```python
from build123d import *

# Parameters (mm, degrees)
SKETCH1_R           = 1.699999809
SKETCH1_R_2         = 1.70000044
BOSS_EXTRUDE1_DEPTH = 5
CHAMFER1_SIZE       = 1.5


with BuildPart() as part:
    # Sketch1 → Boss-Extrude1 (new body)
    with BuildSketch(Plane.XY):
        with BuildLine():
            Line((34.170001984, 18.130024456), (34.170001984, 8.129999593))
            ThreePointArc((34.170001984, 8.129999593), (31.826856233, 2.473145343), (26.170001984, 0.129999593))
            Line((26.170001984, 0.129999593), (8.170027525, 0.129999593))
            ThreePointArc((8.170027525, 0.129999593), (2.513173276, 2.473145343), (0.170027525, 8.129999593))
            Line((0.170027525, 8.129999593), (0.170027525, 18.130024456))
            ThreePointArc((0.170027525, 18.130024456), (2.513173276, 23.786878706), (8.170027525, 26.130024456))
            Line((8.170027525, 26.130024456), (26.170001984, 26.130024456))
            ThreePointArc((26.170001984, 26.130024456), (31.826856233, 23.786878706), (34.170001984, 18.130024456))
        make_face()
        with Locations((17.17000103, 3.630000114)):
            Circle(SKETCH1_R, mode=Mode.SUBTRACT)
        with Locations((17.170001507, 22.630000114)):
            Circle(SKETCH1_R_2, mode=Mode.SUBTRACT)
        with BuildLine():
            Line((30.170001984, 15.629999161), (29.170001984, 15.629999161))
            ThreePointArc((29.170001984, 15.629999161), (28.816448593, 15.77644577), (28.670001984, 16.129999161))
            Line((28.670001984, 16.129999161), (28.670001984, 18.879999161))
            ThreePointArc((28.670001984, 18.879999161), (28.523555374, 19.233552551), (28.170001984, 19.379999161))
            Line((28.170001984, 19.379999161), (6.17000103, 19.379999161))
            ThreePointArc((6.17000103, 19.379999161), (5.816447639, 19.233552551), (5.67000103, 18.879999161))
            Line((5.67000103, 18.879999161), (5.67000103, 7.379999638))
            ThreePointArc((5.67000103, 7.379999638), (5.816447639, 7.026446247), (6.17000103, 6.879999638))
            Line((6.17000103, 6.879999638), (28.170001984, 6.879999638))
            ThreePointArc((28.170001984, 6.879999638), (28.523555374, 7.026446247), (28.670001984, 7.379999638))
            Line((28.670001984, 7.379999638), (28.670001984, 10.130000114))
            ThreePointArc((28.670001984, 10.130000114), (28.816448593, 10.483553505), (29.170001984, 10.630000114))
            Line((29.170001984, 10.630000114), (30.170001984, 10.630000114))
            ThreePointArc((30.170001984, 10.630000114), (30.523555374, 10.776446724), (30.670001984, 11.130000114))
            Line((30.670001984, 11.130000114), (30.670001984, 15.129999161))
            ThreePointArc((30.670001984, 15.129999161), (30.523555374, 15.483552551), (30.170001984, 15.629999161))
        make_face(mode=Mode.SUBTRACT)
    extrude(amount=BOSS_EXTRUDE1_DEPTH)

    # Chamfer1
    chamfer1_edges = [part.edges().sort_by_distance(p)[0] for p in [
        (15.470001221, 3.630000114, 5),
        (15.470001067, 22.630000114, 5),
    ]]
    chamfer(chamfer1_edges, length=CHAMFER1_SIZE)


solid = part.part
```
CAD build for the part. Positions are in the model's coordinates, mm. A direction names the side the tool comes from. Coordinates: 2 decimals unless noted, no trailing zeros. Order: outer loops, then holes, each group sorted by start corner. A loop starts at its lowest first (then second) coordinate and runs counter-clockwise, first axis right, second up. Notation, with made-up numbers: M -1,-3 L 10,-3 A21 cw 10,4 Z; hole C -15,-21 d8. An arc over 180 degrees is marked long. Write each question's results on one line, items separated by ' | '. Start each with the question number.
Q1. Drill centre lines: probe 1 along Y at (x, z) = (20, 2.85); probe 2 along X at (y, z) = (8.75, 0.95); probe 3 along Y at (x, z) = (16.5, 4.2). Where is each one in solid material? Low to high. Write a range as from..to.
Q2. Cut at D-D (z = 2.75). List the corners of the cut face in (x, y), then the cut area to 3 significant figures.
Q3. Cut at A-A (x = 9). List the corners of the cut face in (y, z), then the cut area to 3 significant figures.
Q4. Cut at B-B (y = 22.63). List the corners of the cut face in (x, z).
Q5. Cut at C-C (z = 4.3). List the corners of the cut face in (x, y).
Q6. Which spindle directions (+Z, -Z, +X, -X, +Y, -Y) get a long thin tool onto all of the face, cutting with end or side? Do faces 1 (the flat face through (30, 15.63, 2)), 2 (the flat face through (34.17, 13, 2)). Say none if no direction does.
Q7. Pull direction Y, two halves, no side cores. Call faces 3 (the conical face through (15, 4, 4)), 4 (the cylindrical face through (31.889, 2.536, 2.465)), 5 (the flat face through (0.17, 13, 2)): +Y half, -Y half, draft (parallel to the pull), parting line (faces both ways), or undercut.
Q8. Flat gauge pins, fed straight in: P1, Ø1.1, axis at x = 29.5, z = 1.5, coming from the -Y side; P2, Ø1.5, axis at y = 22.5, z = 2, coming from the -X side. Where does each tip first touch, or does it go through?
Found:
1) probe 1: 0.13..6.88, 19.38..26.13 | probe 2: 0.17..5.67, 28.67..34.17 | probe 3: 0.13..1.33, 5.93..6.88, 19.38..20.33, 24.93..26.13
2) outline: M 0.17,8.13 A8 ccw 8.17,0.13 L 26.17,0.13 A8 ccw 34.17,8.13 L 34.17,18.13 A8 ccw 26.17,26.13 L 8.17,26.13 A8 ccw 0.17,18.13 Z; hole M 5.67,7.38 A0.5 ccw 6.17,6.88 L 28.17,6.88 A0.5 ccw 28.67,7.38 L 28.67,10.13 A0.5 cw 29.17,10.63 L 30.17,10.63 A0.5 ccw 30.67,11.13 L 30.67,15.13 A0.5 ccw 30.17,15.63 L 29.17,15.63 A0.5 cw 28.67,16.13 L 28.67,18.88 A0.5 ccw 28.17,19.38 L 6.17,19.38 A0.5 ccw 5.67,18.88 Z; hole C 17.17,3.63 d3.4; hole C 17.17,22.63 d3.4 | area: 514 mm²
3) outline: M 0.13,0 L 6.88,0 L 6.88,5 L 0.13,5 Z; M 19.38,0 L 26.13,0 L 26.13,5 L 19.38,5 Z | area: 67.5 mm²
4) outline: M 1.56,0 L 15.47,0 L 15.47,3.5 L 13.97,5 L 1.56,5 Z; M 18.87,0 L 32.78,0 L 32.78,5 L 20.37,5 L 18.87,3.5 Z
5) outline: M 0.17,8.13 A8 ccw 8.17,0.13 L 26.17,0.13 A8 ccw 34.17,8.13 L 34.17,18.13 A8 ccw 26.17,26.13 L 8.17,26.13 A8 ccw 0.17,18.13 Z; hole M 5.67,7.38 A0.5 ccw 6.17,6.88 L 28.17,6.88 A0.5 ccw 28.67,7.38 L 28.67,10.13 A0.5 cw 29.17,10.63 L 30.17,10.63 A0.5 ccw 30.67,11.13 L 30.67,15.13 A0.5 ccw 30.17,15.63 L 29.17,15.63 A0.5 cw 28.67,16.13 L 28.67,18.88 A0.5 ccw 28.17,19.38 L 6.17,19.38 A0.5 ccw 5.67,18.88 Z; hole C 17.17,3.63 d5; hole C 17.17,22.63 d5
6) face 1: +Z, -Z | face 2: +Z, -Z, +X, +Y, -Y
7) face 3: undercut | face 4: -Y half | face 5: draft
8) P1: y = 0.63 | P2: x = 1.04
